from build123d import *

# Parameters (mm, degrees)
SKETCH1_W           = 359.918
SKETCH1_H           = 262.89
BOSS_EXTRUDE1_DEPTH = 12.446
SKETCH5_R           = 5
CUT_EXTRUDE1_DEPTH  = 6.223


with BuildPart() as part:
    # Sketch1 → Boss-Extrude1 (new body, symmetric)
    with BuildSketch(Plane(origin=(0, 0, 0), x_dir=(1, 0, 0), z_dir=(0, 1, 0))):
        Rectangle(SKETCH1_W, SKETCH1_H)
    extrude(amount=BOSS_EXTRUDE1_DEPTH, both=True)

    # Sketch5 → Cut-Extrude1 (cut)
    with BuildSketch(Plane(origin=(0, 12.446, 0), x_dir=(1, 0, 0), z_dir=(0, 1, 0))):
        with Locations((-150, 100)):
            Circle(SKETCH5_R)
        with Locations((150, 100)):
            Circle(SKETCH5_R)
        with Locations((150, -100)):
            Circle(SKETCH5_R)
        with Locations((-150, -100)):
            Circle(SKETCH5_R)
    extrude(amount=-CUT_EXTRUDE1_DEPTH, mode=Mode.SUBTRACT)


solid = part.part
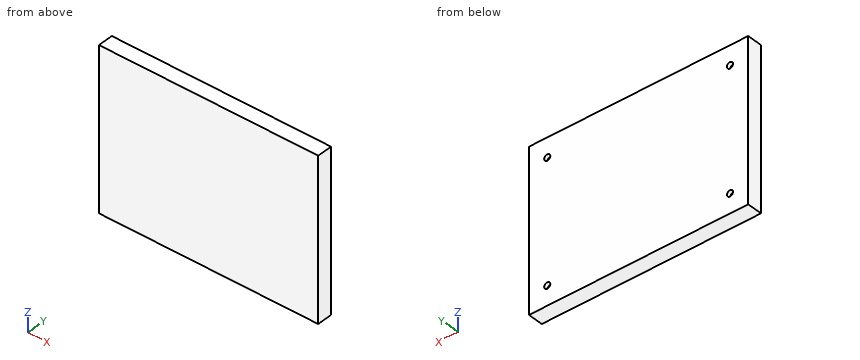
Check sheet for the modelled part. Datum: model origin and axes. Units: mm. Round coordinates to 2 decimals unless told otherwise and drop trailing zeros. Loops run counter-clockwise (first coordinate to the right, second up) from the corner with the lowest first, then second, coordinate; pieces in that order, holes last.
1. Scan lines: probe 1 along X at (y, z) = (7.5, -100); probe 2 along Z at (x, y) = (150, 11) (3 decimals). Record each from-to range of solid material in increasing order.
2. Gauge pin test, flat ends, axial feed: pin 1 Ø11 at (x, z) = (-151.5, -97.5) entering from +Y; pin 2 Ø3 at (x, z) = (152.5, -101.5) entering from +Y. Record the tip position at first contact, or that the pin passes through.
3. Sectioned sample at A-A on x = 150. Record the boundary of the cut face in (y, z) (3 decimals), and give its area (3 significant figures).
Recorded:
1. probe 1: x = -179.96 to -155, -145 to 145, 155 to 179.96
1. probe 2: z = -131.445 to -105, -95 to 95, 105 to 131.445
2. pin 1: stops at y = 12.45
2. pin 2: stops at y = 6.22
3. outline: (-12.446, -131.445) - (12.446, -131.445) - (12.446, -105) - (6.223, -105) - (6.223, -95) - (12.446, -95) - (12.446, 95) - (6.223, 95) - (6.223, 105) - (12.446, 105) - (12.446, 131.445) - (-12.446, 131.445) - close
3. area: 6,420 mm2
